```python
from build123d import *

# Parameters (mm, degrees)
SKETCH1_W                = 170
SKETCH1_H                = 170
BOSS_EXTRUDE1_DEPTH      = 2
F_6_CLEARANCE_HOLE1_D    = 3.7973
SKETCH5_W                = 19
SKETCH5_H                = 27
BOSS_EXTRUDE2_DEPTH      = 31.5
SKETCH6_W                = 19.5
SKETCH6_H                = 28.5
SKETCH6_W_2              = 17.25
SKETCH6_H_2              = 42
BOSS_EXTRUDE3_DEPTH      = 27
SKETCH7_W                = 19.2
SKETCH7_H                = 19.2
BOSS_EXTRUDE4_DEPTH      = 30
SKETCH8_W                = 2
SKETCH8_H                = 25
SKETCH8_W_2              = 1.1
CUT_EXTRUDE1_DEPTH       = 160
SKETCH9_W                = 31
SKETCH9_H                = 11
BOSS_EXTRUDE5_DEPTH      = 6
BOSS_EXTRUDE5_DEPTH_BACK = 4.2


with BuildPart() as part:
    # Sketch1 → Boss-Extrude1 (new body)
    with BuildSketch(Plane(origin=(0, 0, 0), x_dir=(1, 0, 0), z_dir=(0, 1, 0))):
        Rectangle(SKETCH1_W, SKETCH1_H)
    extrude(amount=BOSS_EXTRUDE1_DEPTH)

    # #6 Clearance Hole1 (through all)
    with Locations(Plane(origin=(-78.65, 2, -74.84), x_dir=(0, 0, 1), z_dir=(0, 1, 0))):
        with Locations((0, 0), (154.94, 0), (154.94, 157.48), (22.86, 157.48)):
            Hole(F_6_CLEARANCE_HOLE1_D / 2)

    # Sketch5 → Boss-Extrude2 (add)
    with BuildSketch(Plane(origin=(0, 2, 0), x_dir=(1, 0, 0), z_dir=(0, 1, 0))):
        with Locations((70.2, 71.5)):
            Rectangle(SKETCH5_W, SKETCH5_H)
    extrude(amount=BOSS_EXTRUDE2_DEPTH)

    # Sketch6 → Boss-Extrude3 (add)
    with BuildSketch(Plane(origin=(0, 2, 0), x_dir=(1, 0, 0), z_dir=(0, 1, 0))):
        with Locations((3.7, 70.75)):
            Rectangle(SKETCH6_W, SKETCH6_H)
        with Locations((-19.275, 64)):
            Rectangle(SKETCH6_W_2, SKETCH6_H_2)
    extrude(amount=BOSS_EXTRUDE3_DEPTH)

    # Sketch7 → Boss-Extrude4 (add)
    with BuildSketch(Plane(origin=(0, 2, 0), x_dir=(1, 0, 0), z_dir=(0, 1, 0))):
        with Locations((-41, 64.4)):
            Rectangle(SKETCH7_W, SKETCH7_H)
    extrude(amount=BOSS_EXTRUDE4_DEPTH)

    # Sketch8 → Cut-Extrude1 (cut, through all)
    with BuildSketch(Plane(origin=(0, 0, -74), x_dir=(-1, 0, 0), z_dir=(0, 0, -1))):
        with Locations((33.75, 19.5)):
            Rectangle(SKETCH8_W, SKETCH8_H)
        with Locations((37.1, 19.5)):
            Rectangle(SKETCH8_W, SKETCH8_H)
        with Locations((50.05, 19.5)):
            Rectangle(SKETCH8_W_2, SKETCH8_H)
        with Locations((40.45, 19.5)):
            Rectangle(SKETCH8_W, SKETCH8_H)
        with Locations((47.15, 19.5)):
            Rectangle(SKETCH8_W, SKETCH8_H)
        with Locations((43.8, 19.5)):
            Rectangle(SKETCH8_W, SKETCH8_H)
    extrude(amount=-CUT_EXTRUDE1_DEPTH, mode=Mode.SUBTRACT)

    # Sketch9 → Boss-Extrude5 (add, two sides)
    with BuildSketch(Plane(origin=(0, 0, -85), x_dir=(-1, 0, 0), z_dir=(0, 0, -1))) as boss_extrude5_sk:
        with Locations((47.9, 7.5)):
            Rectangle(SKETCH9_W, SKETCH9_H)
    extrude(amount=BOSS_EXTRUDE5_DEPTH)
    extrude(boss_extrude5_sk.sketch, amount=-BOSS_EXTRUDE5_DEPTH_BACK)


solid = part.part
```
Could you check a few things on this model? Use its own coordinates, in mm. A direction names the side the tool comes from. Round coordinates to 2 decimals unless told otherwise and drop trailing zeros. Order: outer loops, then holes, each group sorted by start corner. A loop starts at its lowest first (then second) coordinate and runs counter-clockwise, first axis right, second up. Notation, with made-up numbers: (71, -17.75) -> (118, -17.75) arc R12 ccw to (118, 2.25) -> close; hole circle Ø8 at (47, -11.75). An arc over 180 degrees is marked (long way). One line per question, with ' | ' between items.
Q1. I'm going to push flat-ended pins straight in: pin 1 (12 mm diameter, centred on y = 8.5, z = 12, fed in from +X); pin 2 (15.5 mm diameter, centred on y = 19.5, z = -65.5, fed in from -X); pin 3 (10 mm diameter, centred on x = 56.5, z = 45, fed in from +Y); pin 4 (9.5 mm diameter, centred on y = 21.5, z = -68.5, fed in from +X). Where does each tip first touch, or does it pass through?
Computed values:
pin 1: through | pin 2: x = -49.5 | pin 3: y = 2 | pin 4: x = 79.7
Q2. We'd pull the mould along X, two halves only. Please class faces 6 (the face through (-31.4, 17, -64)), 7 (the face through (-48, 13, -86)), 8 (the face through (-39.45, 19, -65)): released by +X, released by -X, zero draft, split by the parting line, or undercut.
Computed values:
face 6: undercut | face 7: zero draft | face 8: undercut
Q3. If I drill on line 1 (Z direction, x = -78.65, y = 1.5); line 2 (X direction, y = 0.65, z = -51.98); line 3 (Y direction, x = 20, z = 32), over which ranges is the centre line in solid material (lowest first)? Write a range as from..to.
Computed values:
line 1: -85..-76.74, -72.94..78.2, 82..85 | line 2: -85..76.93, 80.73..85 | line 3: 0..2
Q4. If we section it at A-A on y = 15.5: Give the number of separate pieces and of enclosed holes in the cut face, plus the area to 3 significant figures.
Computed values:
separate pieces: 9 | enclosed holes: 0 | area: 1,950 mm²
Q5. If we section it at D-D on x = -67: Write out the boundary of the cut face in (y, z).
Computed values:
outline: (0, -85) -> (2, -85) -> (2, 85) -> (0, 85) -> close
Q6. If we section it at C-C on z = -38.5: Write out the boundary of the cut face in (x, y).
Computed values:
outline: (-85, 0) -> (85, 0) -> (85, 2) -> (-85, 2) -> close
Q7. If we section it at B-B on x = -25.5: Write out the boundary of the cut face in (y, z), plus the area to 3 significant figures.
Computed values:
outline: (0, -85) -> (29, -85) -> (29, -43) -> (2, -43) -> (2, 85) -> (0, 85) -> close | area: 1,470 mm²
Q8. Which directions (+Z, -Z, +X, -X, +Y, -Y) give clear straight access to the entire face, cutting with the end or side of a thin tool? Please do faces 1 (the face through (-42.8, 19, -65)), 2 (the face through (-48, 2, -88)), 3 (the face through (-27.9, 15, -64)), 4 (the face through (-1, 0, -1)), 5 (the face through (4, 15, -56.5)).
Computed values:
face 1: +Z, +Y | face 2: -Z, +X, -X, -Y | face 3: +Z, -Z, +Y | face 4: +Z, -Z, +X, -X, -Y | face 5: +Z, +X, +Y
